Could you check a few things on this drawing? It's one solid part, dimensions in mm from its lowest x, y, z. Give positions to 0.01 mm unless a question says otherwise; leave off trailing zeros. Order: outer loops, then holes, each group sorted by start corner. A loop starts at its lowest first (then second) coordinate and runs counter-clockwise, first axis right, second up. Notation, with made-up numbers: M -24,-36 L -8,-36 A19 cw -8,-20 Z; hole C 21,76.5 d3. An arc over 180 degrees is marked long. One line per item, written item: value. Start each with the question number.
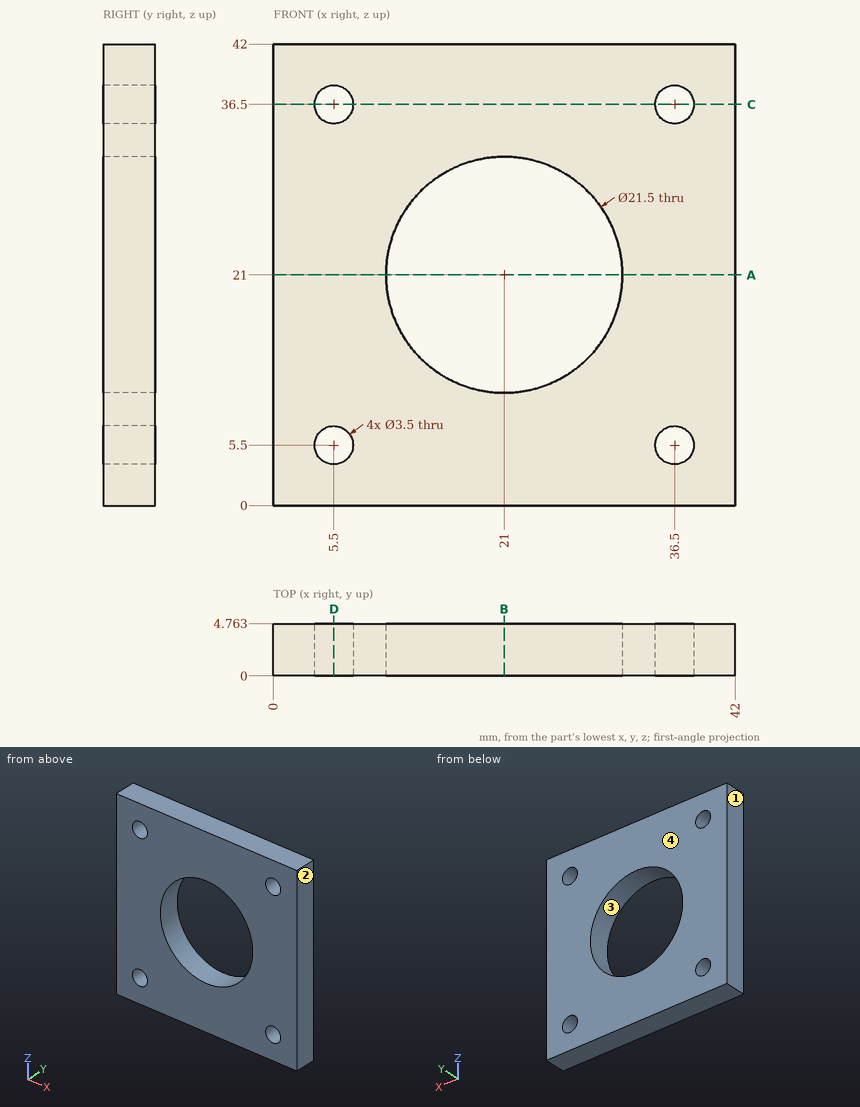
Item 1: Please list where these lines run through material, in increasing order: probe 1 along Z at (x, y) = (36.5, 3.2); probe 2 along X at (y, z) = (1.9, 21); probe 3 along Z at (x, y) = (24, 1.35). Write a range as [from, to].
Item 2: I want a section at D-D on x = 5.5. Write out the boundary of the cut face in (y, z).
Item 3: I want a section at A-A on z = 21. Write out the boundary of the cut face in (x, y).
Item 4: I want a section at B-B on x = 21. Write out the boundary of the cut face in (y, z).
Item 5: I want a section at C-C on z = 36.5. Write out the boundary of the cut face in (x, y), plus the area to 3 significant figures.
Item 6: We'd pull the mould along X, two halves only. Please class the marked faces 1, 2, 3 and 4: +X half, -X half, draft (parallel to the pull), parting line (faces both ways), or undercut.
Item 7: Will this pin go through, and if not, where does the flat tip stop? P1, Ø6, axis at x = 20, z = 26.5, coming from the -Y side.
Answer below:
1. probe 1: z = [0, 3.75], [7.25, 34.75], [38.25, 42]
1. probe 2: x = [0, 10.25], [31.75, 42]
1. probe 3: z = [0, 10.68], [31.32, 42]
2. outline: M 0,0 L 4.76,0 L 4.76,3.75 L 0,3.75 Z; M 0,7.25 L 4.76,7.25 L 4.76,34.75 L 0,34.75 Z; M 0,38.25 L 4.76,38.25 L 4.76,42 L 0,42 Z
3. outline: M 0,0 L 10.25,0 L 10.25,4.76 L 0,4.76 Z; M 31.75,0 L 42,0 L 42,4.76 L 31.75,4.76 Z
4. outline: M 0,0 L 4.76,0 L 4.76,10.25 L 0,10.25 Z; M 0,31.75 L 4.76,31.75 L 4.76,42 L 0,42 Z
5. outline: M 0,0 L 3.75,0 L 3.75,4.76 L 0,4.76 Z; M 7.25,0 L 34.75,0 L 34.75,4.76 L 7.25,4.76 Z; M 38.25,0 L 42,0 L 42,4.76 L 38.25,4.76 Z
5. area: 167 mm²
6. face 1: -X half
6. face 2: +X half
6. face 3: undercut
6. face 4: draft
7. P1: passes through
